Geometry check sheet. Reference: the model listing, model coordinates, mm. Coordinates: 2 decimals unless noted, no trailing zeros. Loops run counter-clockwise (first coordinate to the right, second up) from the corner with the lowest first, then second, coordinate; pieces in that order, holes last.
from build123d import *

# Parameters (mm, degrees)
SKETCH1_R           = 3.3
BOSS_EXTRUDE1_DEPTH = 3.175
FILLET1_R           = 2.54


with BuildPart() as part:
    # Sketch1 → Boss-Extrude1 (new body)
    with BuildSketch(Plane(origin=(0, 0, 0), x_dir=(1, 0, 0), z_dir=(0, 1, 0))):
        with BuildLine():
            Line((-48.70903707, -102.985419006), (-49.602131042, -106.032221946))
            Line((-49.602131042, -106.032221946), (-55.631977257, -126.603129099))
            Line((-55.631977257, -126.603129099), (-12.618209883, -129.313914375))
            Line((-12.618209883, -129.313914375), (-6.890929076, -109.775213464))
            Line((-6.890929076, -109.775213464), (-5.88465666, -106.342300635))
            ThreePointArc((-5.88465666, -106.342300635), (-27.452664405, -106.651653953), (-48.70903707, -102.985419006))
        make_face()
        with Locations(Location((-39.544579652, -121.411764721, 0), (0, 0, 270))):
            Circle(SKETCH1_R, mode=Mode.SUBTRACT)
    extrude(amount=BOSS_EXTRUDE1_DEPTH)

    # Fillet1
    fillet1_edges = [part.edges().sort_by_distance(p)[0] for p in [
        (-5.88465666, 1.5875, 106.342300635),
        (-12.618209883, 1.5875, 129.313914375),
        (-55.631977257, 1.5875, 126.603129099),
        (-48.70903707, 1.5875, 102.985419006),
    ]]
    fillet(fillet1_edges, radius=FILLET1_R)


solid = part.part
(1) Sectioned sample at B-B on x = -40. Record the cut outline in (y, z) (3 decimals), and give its area (3 significant figures).
Findings:
outline: (0, 104.979) - (3.175, 104.979) - (3.175, 118.143) - (0, 118.143) - close; (0, 124.68) - (3.175, 124.68) - (3.175, 127.588) - (0, 127.588) - close
area: 51.0 mm2
(2) Scan lines: L1, parallel to Z at x = -39.5, y = 2.6; L2, parallel to Z at x = -38, y = 2.5; L3, parallel to X at y = 2.5, z = 119. Record each from-to range of solid material in increasing order.
Findings:
L1: z = 105.07 to 118.11, 124.71 to 127.62
L2: z = 105.34 to 118.5, 124.33 to 127.71
L3: x = -53.4 to -41.8, -37.29 to -9.59
(3) Sectioned sample at A-A on z = 120.75. Record the cut outline in (x, y) (3 decimals).
Findings:
outline: (-53.916, 0) - (-42.778, 0) - (-42.778, 3.175) - (-53.916, 3.175) - close; (-36.312, 0) - (-10.108, 0) - (-10.108, 3.175) - (-36.312, 3.175) - close
(4) Sectioned sample at D-D on z = 113.5. Record the cut outline in (x, y) (3 decimals).
Findings:
outline: (-51.791, 0) - (-7.983, 0) - (-7.983, 3.175) - (-51.791, 3.175) - close
(5) Sectioned sample at C-C on x = -11. Record the cut outline in (y, z) (3 decimals).
Findings:
outline: (0, 106.778) - (3.175, 106.778) - (3.175, 123.793) - (0, 123.793) - close
(6) Gauge pin test, flat end, axial feed: pin 1 Ø1 at (y, z) = (1.5, 123) entering from +X. Record the tip position at first contact, or that the pin passes through.
Findings:
pin 1: stops at x = -10.62
